Check sheet for the modelled part. Datum: model origin and axes. Units: mm. Face numbers are marked on the shaded views. Round coordinates to 2 decimals unless told otherwise and drop trailing zeros. Loops run counter-clockwise (first coordinate to the right, second up) from the corner with the lowest first, then second, coordinate; pieces in that order, holes last. Notation, with made-up numbers: (86.25, -29) - (112.25, -29) arc R24 cw to (112.25, -11) - close; hole circle Ø8 at (-15.75, 77). An arc over 180 degrees is marked (long way). Put each result on its own line as item: value. Start each with the question number.
Item 1: Section check B-B, the plane z = 0. Record the cut outline in (x, y).
Item 2: Material ranges on line 1 along Z through (x, y) = (0, 3); line 2 along X through (y, z) = (3.9, 0); line 3 along X through (y, z) = (3.75, -1.5), recorded low to high.
Item 3: Section check A-A, the plane x = 0. Record the cut outline in (y, z).
Item 4: Draft check along Z on the marked faces 1, 2 and 3. Enter one of: pulls with the +Z half, pulls with the -Z half, needs draft (parallel to the pull), parting line crosses it, or undercut.
Autodesk Inventor part; units mm, degrees
ref_plane "YZ Plane" through (0, 0, 0) normal (1, 0, 0) x (0, 1, 0)
ref_plane "XZ Plane" through (0, 0, 0) normal (0, 1, 0) x (-1, 0, 0)
ref_plane "XY Plane" through (0, 0, 0) normal (0, 0, 1) x (1, 0, 0)
sketch "Náčrt2" plane through (0, 0, 0) normal (0, 1, 0) x (-1, 0, 0)
  line L0 (32.5, 17.5) -> (-32.5, 17.5)
  line L1 (-32.5, 17.5) -> (-32.5, -17.5)
  line L2 (-32.5, -17.5) -> (32.5, -17.5)
  line L3 (32.5, -17.5) -> (32.5, 17.5)
  point P0 (0, 0)
  point P1 (32.5, 0)
  point P2 (0, 17.5)
  dimension "d0" = 65
  dimension "d1" = 35
extrude "Vysunutí1" add sketch "Náčrt2" along normal blind 6
chamfer "Zkosení3" distance 2 angle 45 2 edges at (-32.5, 6, 0) (32.5, 6, 0)
sketch "Náčrt6" plane through (0, 6, 0) normal (0, 1, 0) x (1, 0, 0)
  point P0 (0, 0)
hole "Díra1" at (0, 6, 0) direction (0, -1, 0) diameter 6.647 end through all
chamfer "Zkosení4" distance 0.4 angle 45 1 edges at (0, 6, -3.3235)
equation "\"PoloměrOhybu\" = Tloušťka"
equation "\"ŠířkaVýštipu\" = Tloušťka"
equation "\"HloubkaVýštipu\" = 0.5 * Tloušťka"
equation "\"MinimálníZbytek\" = 2 * Tloušťka"
equation "\"PřechodovýPoloměr\" = PoloměrOhybu"
equation "\"VelikostJacobihoPoloměru\" = PoloměrOhybu"
equation "\"VelikostMezery\" = Tloušťka"
properties part number "DD_KVD_004_04_B" material "Nerezová ocel"
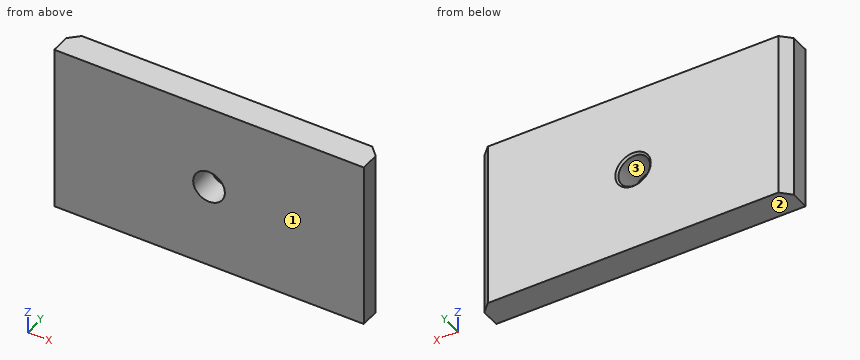
Check result:
1. outline: (-32.5, 0) - (-3.32, 0) - (-3.32, 5.6) - (-3.72, 6) - (-30.5, 6) - (-32.5, 4) - close; (3.32, 0) - (32.5, 0) - (32.5, 4) - (30.5, 6) - (3.72, 6) - (3.32, 5.6) - close
2. line 1: -17.5 to -3.32, 3.32 to 17.5
2. line 2: -32.5 to -3.32, 3.32 to 32.5
2. line 3: -32.5 to -2.97, 2.97 to 32.5
3. outline: (0, -17.5) - (6, -17.5) - (6, -3.72) - (5.6, -3.32) - (0, -3.32) - close; (0, 3.32) - (5.6, 3.32) - (6, 3.72) - (6, 17.5) - (0, 17.5) - close
4. face 1: needs draft
4. face 2: pulls with the -Z half
4. face 3: undercut
